Verification items for this drawing (mm, ordinates from the low corner). Coordinates: 2 decimals unless noted, no trailing zeros. Order: outer loops, then holes, each group sorted by start corner. A loop starts at its lowest first (then second) coordinate and runs counter-clockwise, first axis right, second up. Notation, with made-up numbers: M 17.25,12 L 56.25,12 A23 cw 56.25,51 Z; hole C -11,51 d7. An arc over 180 degrees is marked long. Answer as a JSON object with one key per item and string values. Group by question number.
(1) Cross-section at B-B (z = 90). Enter the section's corners in (x, y), plus the area to 3 significant figures.
(2) Material ranges on line 1 (X direction, y = 1.75, z = 90); line 2 (X direction, y = 2, z = 15); line 3 (Z direction, x = 70.95, y = 3), recorded low to high.
(3) Cross-section at C-C (x = 123.5). Enter the section's corners in (y, z).
(4) Cross-section at D-D (z = 113). Enter the section's corners in (x, y).
(5) Cross-section at A-A (y = 4). Count the separate pieces of the cut face and the enclosed holes in it, plus the area to 3 significant figures.
(6) Gauge pin test, flat ends, axial feed: pin 1 Ø1.5 at (x, y) = (55.5, 5) entering from -Z; pin 2 Ø4 at (x, y) = (80.5, 3) entering from +Z. Record the tip position at first contact, or that the pin passes through.
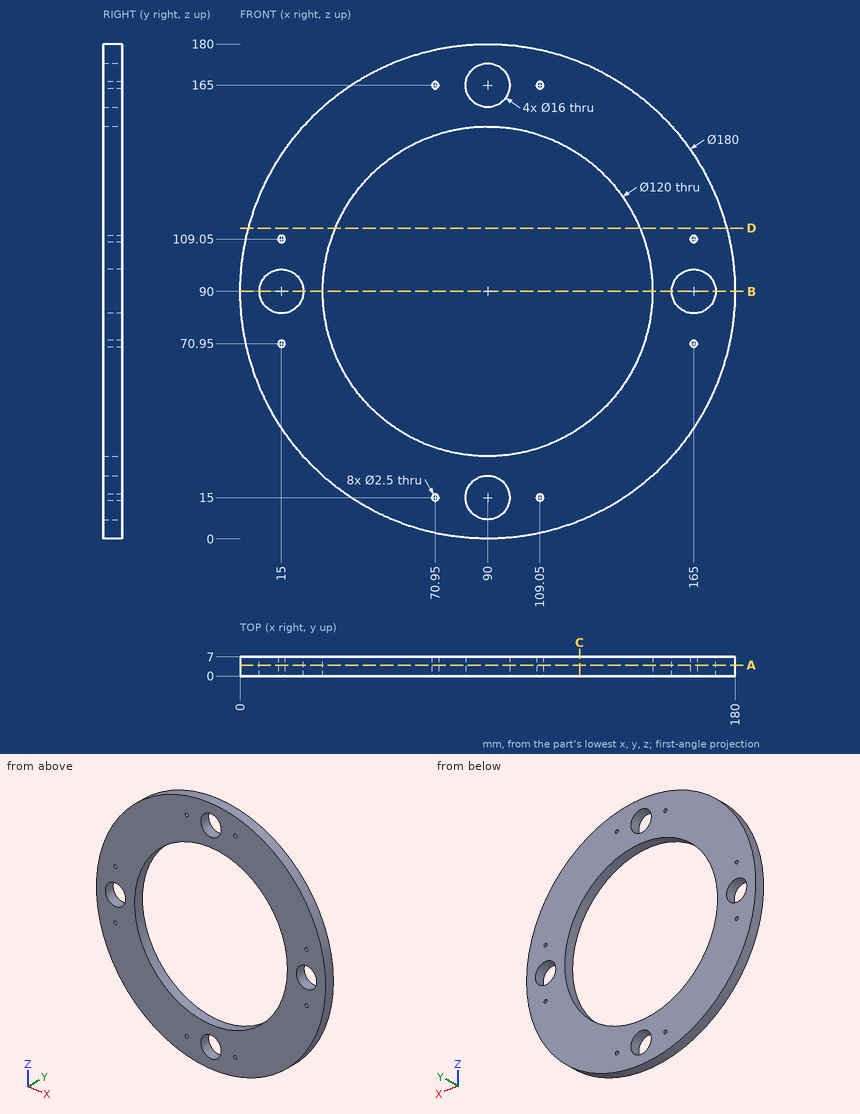
Taken from the geometry:
{
 "1": {"outline": "M 0,0 L 7,0 L 7,7 L 0,7 Z; M 23,0 L 30,0 L 30,7 L 23,7 Z; M 150,0 L 157,0 L 157,7 L 150,7 Z; M 173,0 L 180,0 L 180,7 L 173,7 Z", "area": "196 mm²"},
 "2": {"line 1": "x = 0 to 7, 23 to 30, 150 to 157, 173 to 180", "line 2": "x = 40.25 to 69.7, 72.2 to 82, 98 to 107.8, 110.3 to 139.75", "line 3": "z = 2.04 to 13.75, 16.25 to 33.1, 146.9 to 163.75, 166.25 to 177.96"},
 "3": {"outline": "M 0,6.47 L 7,6.47 L 7,40.22 L 0,40.22 Z; M 0,139.78 L 7,139.78 L 7,173.53 L 0,173.53 Z"},
 "4": {"outline": "M 2.99,0 L 34.58,0 L 34.58,7 L 2.99,7 Z; M 145.42,0 L 177.01,0 L 177.01,7 L 145.42,7 Z"},
 "5": {"separate pieces": "1", "enclosed holes": "13", "area": "13,300 mm²"},
 "6": {"pin 1": "stops at z = 6.57", "pin 2": "stops at z = 179.69"}
}
